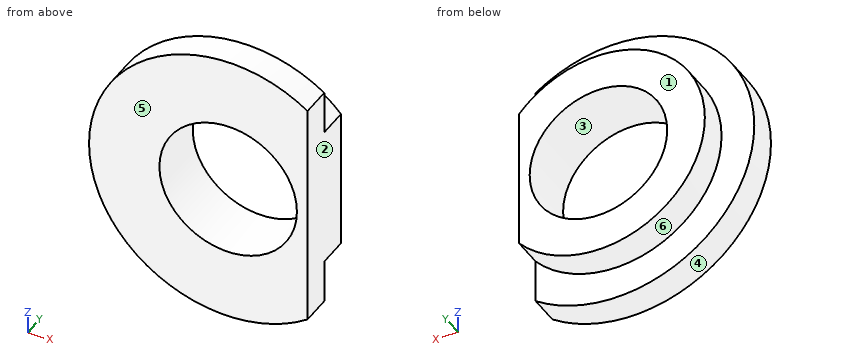
Autodesk Inventor part; units mm, degrees
ref_plane "YZ Plane" through (0, 0, 0) normal (1, 0, 0) x (0, 1, 0)
ref_plane "XZ Plane" through (0, 0, 0) normal (0, 1, 0) x (-1, 0, 0)
ref_plane "XY Plane" through (0, 0, 0) normal (0, 0, 1) x (1, 0, 0)
sketch "Sketch1" plane through (0, 0, 0) normal (0, 1, 0) x (-1, 0, 0)
  circle A0 centre (0, 0) radius 5.5626
  dimension "d0" = 11.1252
extrude "Extrusion1" add sketch "Sketch1" along normal blind 1.2192
sketch "Sketch2" plane through (0, 1.2192, 0) normal (0, 1, 0) x (1, 0, 0)
  circle A0 centre (0, 0) radius 4.2545
  dimension "d3" = 8.509
extrude "Extrusion2" add sketch "Sketch2" along normal blind 1.2192
sketch "Sketch3" plane through (0, 2.4384, 0) normal (0, 1, 0) x (1, 0, 0)
  circle A0 centre (0, 0) radius 2.75
  dimension "d6" = 5.5
extrude "Extrusion3" cut sketch "Sketch3" against normal blind 4.064
sketch "Sketch4" plane through (0, 2.4384, 0) normal (0, 1, 0) x (1, 0, 0)
  line L0 (15.9461, 14.0442) -> (3.175, 14.0442)
  line L1 (3.175, 14.0442) -> (3.175, -15.9032)
  line L2 (3.175, -15.9032) -> (15.9461, -15.9032)
  line L3 (15.9461, -15.9032) -> (15.9461, 14.0442)
  point P0 (0, 0)
  dimension "d9" = 3.175
extrude "Extrusion4" cut sketch "Sketch4" against normal blind 4.064
properties part number "Spring Clamp Small"
The model under review builds one solid part; all positions refer to its coordinate system, in mm. Face numbers are marked on the shaded views. A direction names the side the tool comes from. Round coordinates to 2 decimals unless told otherwise and drop trailing zeros. Write each loop counter-clockwise with the first axis right and the second up, starting at its lowest first coordinate (ties: lowest second). Pieces come first, ordered by that corner, then holes. Notation, with made-up numbers: M 62.25,51.25 L 72.25,51.25 A27 cw 72.25,75.25 Z; hole C 32.5,-36.5 d4. An arc over 180 degrees is marked long. Answer as CSV lines item,"result". Start each with the question number.
Q1. Consider section D-D, the plane y = 1.1. Give the boundary of the cut face in (x, z) (3 decimals), then the cut area to 3 significant figures.
Q2. Wall thickness on line 1 along X through (y, z) = (1, 0) (3 decimals); line 2 along Z through (x, y) = (0, 1.3); line 3 along Y through (x, z) = (0.75, -4.25): over which ranges is each line inside the solid? List them lowest first.
Q3. Consider section B-B, the plane x = 0. Give the boundary of the cut face in (y, z).
Q4. Consider section C-C, the plane x = -4. Give the boundary of the cut face in (y, z).
Q5. Clearance check with a flat-ended pin moving along its axis: P1, Ø2, axis at x = 2, z = 1.5, coming from the +Y side. State where the tip first meets the part, or that it passes through.
Q6. Tool access review of the marked faces 5 and 6: name each direction out of +Z, -Z, +X, -X, +Y, -Y from which nothing blocks a thin tool from reaching the whole face with its end or side.
Q7. The part is to be moulded in two halves that separate along X. For the marked faces 1, 2, 3 and 4, say which applies: +X half, -X half, draft (parallel to the pull), parting line (faces both ways), or undercut.
Result set:
1,outline,"M 3.175,-4.567 L 3.175,4.567 A5.563 ccw long Z; hole C 0,0 d5.5"
1,area,"58.1 mm²"
2,line 1,"x = -5.563 to -2.75, 2.75 to 3.175"
2,line 2,"z = -4.25 to -2.75, 2.75 to 4.25"
2,line 3,"y = 0 to 1.22"
3,outline,"M 0,-5.56 L 1.22,-5.56 L 1.22,-4.25 L 2.44,-4.25 L 2.44,-2.75 L 0,-2.75 Z; M 0,2.75 L 2.44,2.75 L 2.44,4.25 L 1.22,4.25 L 1.22,5.56 L 0,5.56 Z"
4,outline,"M 0,-3.87 L 1.22,-3.87 L 1.22,-1.45 L 2.44,-1.45 L 2.44,1.45 L 1.22,1.45 L 1.22,3.87 L 0,3.87 Z"
5,P1,"stops at y = 2.44"
6,face 5,"+Z, -Z, +X, -X, -Y"
6,face 6,"+Y"
7,face 1,"draft"
7,face 2,"+X half"
7,face 3,"undercut"
7,face 4,"parting line"
